Source: CAD feature listing. Evaluate the final solid. Frame: model axes, mm. A direction names the side the tool comes from. Give positions to 0.01 mm unless a question says otherwise; leave off trailing zeros. Loops run counter-clockwise (first coordinate to the right, second up) from the corner with the lowest first, then second, coordinate; pieces in that order, holes last. Notation, with made-up numbers: M 32,29.5 L 53,29.5 A27 cw 53,45.5 Z; hole C 49.5,20.5 d11. An arc over 180 degrees is marked long. Put each result on its own line as item: value.
from build123d import *

# Parameters (mm, degrees)
ESTRUSIONE_ESTRUSIONE1_DEPTH   = 5
FORO_PER_VITE_M6_1_D           = 6.6
FORO_PER_VITE_M6_1_CSINK_D     = 6.65
FORO_PER_VITE_M6_1_CSINK_ANGLE = 90
SCHIZZO4_R                     = 26.5
SCHIZZO4_R_2                   = 23.5
ESTRUSIONE_ESTRUSIONE2_DEPTH   = 24
SCHIZZO5_R                     = 11.5
TAGLIO_ESTRUSIONE1_DEPTH       = 5
SMUSSO1_SIZE                   = 0.5


with BuildPart() as part:
    # Schizzo1 → Estrusione-Estrusione1 (new body)
    with BuildSketch(Plane.XY):
        with BuildLine():
            Line((2.4885721, -39.50156014), (20.319683996, -37.803546229))
            ThreePointArc((20.319683996, -37.803546229), (27.963406237, -31.07606674), (30.391301643, -21.187143955))
            Line((30.391301643, -21.187143955), (23.49327463, -2.368382239))
            ThreePointArc((23.49327463, -2.368382239), (21.78857361, 1.396167849), (19.548342312, 4.868804695))
            Line((19.548342312, 4.868804695), (7.275368714, 21.121066322))
            ThreePointArc((7.275368714, 21.121066322), (-2.796248933, 24.425719741), (-12.86786658, 21.121066322))
            Line((-12.86786658, 21.121066322), (-25.140840178, 4.868804695))
            ThreePointArc((-25.140840178, 4.868804695), (-27.381071476, 1.396167849), (-29.085772496, -2.368382239))
            Line((-29.085772496, -2.368382239), (-35.983799509, -21.187143955))
            ThreePointArc((-35.983799509, -21.187143955), (-33.555904103, -31.07606674), (-25.912181862, -37.803546229))
            Line((-25.912181862, -37.803546229), (-8.081069967, -39.50156014))
            ThreePointArc((-8.081069967, -39.50156014), (-2.796248933, -40.00482094), (2.4885721, -39.50156014))
        make_face()
    extrude(amount=ESTRUSIONE_ESTRUSIONE1_DEPTH)

    # Foro per Vite M6-1 (through all)
    with Locations(Plane(origin=(0, 0, 0), x_dir=(-1, 0, 0), z_dir=(0, 0, -1))):
        with Locations((2.796248933, 19.99517906), (29.907132357, -29.00482094), (-24.31463449, -29.00482094)):
            CounterSinkHole(FORO_PER_VITE_M6_1_D / 2, FORO_PER_VITE_M6_1_CSINK_D / 2, counter_sink_angle=FORO_PER_VITE_M6_1_CSINK_ANGLE)

    # Schizzo4 → Estrusione-Estrusione2 (add)
    with BuildSketch(Plane.XY.offset(5)):
        with Locations((-2.796248933, -12.00482094)):
            Circle(SCHIZZO4_R)
        with Locations((-2.796248933, -12.00482094)):
            Circle(SCHIZZO4_R_2, mode=Mode.SUBTRACT)
    extrude(amount=ESTRUSIONE_ESTRUSIONE2_DEPTH)

    # Schizzo5 → Taglio-Estrusione1 (cut)
    with BuildSketch(Plane(origin=(0, 0, 0), x_dir=(-1, 0, 0), z_dir=(0, 0, -1))):
        with Locations((2.796248933, -12.00482094)):
            Circle(SCHIZZO5_R)
    extrude(amount=-TAGLIO_ESTRUSIONE1_DEPTH, mode=Mode.SUBTRACT)

    # Smusso1
    smusso1_edges = [part.edges().sort_by_distance(p)[0] for p in [
        (-29.296248933, -12.00482094, 29),
        (-26.296248933, -12.00482094, 29),
    ]]
    chamfer(smusso1_edges, length=SMUSSO1_SIZE)


solid = part.part
1. Section query B-B (x = -5). State how many separate pieces and enclosed holes the cut face has, plus the area to 3 significant figures.
Found:
separate pieces: 3
enclosed holes: 0
area: 328 mm^2
2. Material intervals for line 1 (Z direction, x = -26, y = -12.5); line 2 (Y direction, x = -10.5, z = 21.5); line 3 (X direction, y = -26, z = 15), sorted ascending. Write a range as from..to.
Found:
line 1: 0..5
line 2: -37.36..-34.21, 10.2..13.35
line 3: -25.3..-21.67, 16.08..19.71
3. Contact query for flat-ended pins moving along their axis: P1, Ø8.5, axis at x = -29.91, y = -29, coming from the +Z side; P2, Ø6, axis at x = -29, z = 19, coming from the -Y side; P3, Ø4, axis at x = 3, z = 3, coming from the -Y side. Output: stop coordinate, or through.
Found:
P1: z = 5
P2: y = -24.8
P3: y = -39.75
4. Draft query along Y for faces 1 (the flat face through (-32.49, -11.65, 2.46)), 2 (the flat face through (20, -20, 29)), 3 (the cylindrical face through (-23.826, -28.13, 16.586)), 4 (the cylindrical face through (27.363, -30.269, 2.547)). Return one class per face: pulls with the +Y half, pulls with the -Y half, needs draft (parallel to the pull), parting line crosses it, or undercut.
Found:
face 1: pulls with the +Y half
face 2: needs draft
face 3: parting line crosses it
face 4: undercut
5. Access query for faces 5 (the flat face through (-17.12, -38.64, 2.46)), 6 (the flat face through (-10, 14, 5)). Directions: +Z, -Z, +X, -X, +Y, -Y. A direction counts if a zero-diameter tool reaches every point of the face in a straight line with its end or side. Return the directions, or none.
Found:
face 5: +Z, -Z, -X, -Y
face 6: +Z
6. Section query A-A (z = 3.75). Output: boundary loops of the cut face in (x, y).
Found:
outline: M -35.98,-21.19 A17 ccw -25.91,-37.8 L -8.08,-39.5 A28 ccw 2.49,-39.5 L 20.32,-37.8 A17 ccw 30.39,-21.19 L 23.49,-2.37 A28 ccw 19.55,4.87 L 7.28,21.12 A17 ccw -12.87,21.12 L -25.14,4.87 A28 ccw -29.09,-2.37 Z; hole C -29.91,-29 d6.6; hole C -2.8,-12 d23; hole C -2.8,20 d6.6; hole C 24.31,-29 d6.6
7. Section query C-C (z = 16.75). Output: boundary loops of the cut face in (x, y), plus the area to 3 significant figures.
Found:
outline: C -2.8,-12 d53; hole C -2.8,-12 d47
area: 471 mm^2
